CAD build for the part. Positions are in the model's coordinates, mm. A direction names the side the tool comes from. Round coordinates to 2 decimals unless told otherwise and drop trailing zeros. Order: outer loops, then holes, each group sorted by start corner. A loop starts at its lowest first (then second) coordinate and runs counter-clockwise, first axis right, second up. Notation, with made-up numbers: (67.25, 49.25) - (75.25, 49.25) arc R21 ccw to (75.25, 66.25) - close; hole circle Ø8 at (29.25, -20). An arc over 180 degrees is marked (long way). Write item = value, one per line.
from build123d import *

# Parameters (mm, degrees)
SKETCH1_W           = 67.3
SKETCH1_H           = 135.4
BOSS_EXTRUDE1_DEPTH = 15.1
FILLET1_R           = 5
FILLET2_R           = 3.75
SKETCH2_W           = 12.2
SKETCH2_H           = 4.45
CUT_EXTRUDE1_DEPTH  = 6
SKETCH3_W           = 8.2
SKETCH3_H           = 3.5
SKETCH3_W_2         = 8
SKETCH3_H_2         = 3.3
CUT_EXTRUDE2_DEPTH  = 3
FILLET3_R           = 3.75
SKETCH4_W           = 8
SKETCH4_H           = 3.3
BOSS_EXTRUDE2_DEPTH = 0.5
FILLET4_R           = 0.2
FILLET5_R           = 0.2
BOSS_EXTRUDE3_DEPTH = 2.1


with BuildPart() as part:
    # Sketch1 → Boss-Extrude1 (new body)
    with BuildSketch(Plane(origin=(0, 0, 0), x_dir=(1, 0, 0), z_dir=(0, 1, 0))):
        with Locations((33.65, 67.7)):
            Rectangle(SKETCH1_W, SKETCH1_H)
    extrude(amount=BOSS_EXTRUDE1_DEPTH)

    # Fillet1
    fillet1_edges = [part.edges().sort_by_distance(p)[0] for p in [
        (0, 7.55, -135.4),
        (67.3, 7.55, -135.4),
        (67.3, 7.55, 0),
        (0, 7.55, 0),
    ]]
    fillet(fillet1_edges, radius=FILLET1_R)

    # Fillet2
    fillet2_edges = [part.edges().sort_by_distance(p)[0] for p in [
        (0, 15.1, -67.7),
        (33.65, 15.1, -135.4),
        (33.65, 15.1, 0),
        (67.3, 15.1, -67.7),
        (1.464466094, 15.1, -1.464466094),
        (65.835533906, 15.1, -1.464466094),
        (65.835533906, 15.1, -133.935533906),
        (1.464466094, 15.1, -133.935533906),
    ]]
    fillet(fillet2_edges, radius=FILLET2_R)

    # Sketch2 → Cut-Extrude1 (cut)
    with BuildSketch(Plane.XY):
        with Locations((17.1, 8.125)):
            Rectangle(SKETCH2_W, SKETCH2_H)
        with Locations((50.2, 8.125)):
            Rectangle(SKETCH2_W, SKETCH2_H)
        with BuildLine():
            Line((30.7, 7.45), (36.6, 7.45))
            ThreePointArc((36.6, 7.45), (37.448528137, 7.801471863), (37.8, 8.65))
            Line((37.8, 8.65), (37.8, 9.15))
            ThreePointArc((37.8, 9.15), (37.448528137, 9.998528137), (36.6, 10.35))
            Line((36.6, 10.35), (30.7, 10.35))
            ThreePointArc((30.7, 10.35), (29.851471863, 9.998528137), (29.5, 9.15))
            Line((29.5, 9.15), (29.5, 8.65))
            ThreePointArc((29.5, 8.65), (29.851471863, 7.801471863), (30.7, 7.45))
        make_face()
    extrude(amount=-CUT_EXTRUDE1_DEPTH, mode=Mode.SUBTRACT)

    # Sketch3 → Cut-Extrude2 (cut)
    with BuildSketch(Plane(origin=(67.3, 0, 0), x_dir=(0, 0, -1), z_dir=(1, 0, 0))):
        with Locations((15.6, 7.6)):
            Rectangle(SKETCH3_W, SKETCH3_H)
        with Locations((15.6, 7.6)):
            Rectangle(SKETCH3_W_2, SKETCH3_H_2, mode=Mode.SUBTRACT)
    extrude(amount=-CUT_EXTRUDE2_DEPTH, mode=Mode.SUBTRACT)

    # Fillet3
    fillet3_edges = [part.edges().sort_by_distance(p)[0] for p in [
        (0, 0, -67.7),
        (33.65, 0, -135.4),
        (67.3, 0, -67.7),
        (33.65, 0, 0),
        (1.464466094, 0, -1.464466094),
        (65.835533906, 0, -1.464466094),
        (65.835533906, 0, -133.935533906),
        (1.464466094, 0, -133.935533906),
    ]]
    fillet(fillet3_edges, radius=FILLET3_R)

    # Sketch4 → Boss-Extrude2 (add)
    with BuildSketch(Plane(origin=(67.3, 0, 0), x_dir=(0, 0, -1), z_dir=(1, 0, 0))):
        with Locations((15.6, 7.6)):
            Rectangle(SKETCH4_W, SKETCH4_H)
    extrude(amount=BOSS_EXTRUDE2_DEPTH)

    # Fillet4
    fillet4_edges = [part.edges().sort_by_distance(p)[0] for p in [
        (66.05, 9.25, -11.6),
        (66.05, 9.25, -19.6),
        (66.05, 5.95, -19.6),
        (66.05, 5.95, -11.6),
    ]]
    fillet(fillet4_edges, radius=FILLET4_R)

    # Fillet5
    fillet5_edges = [part.edges().sort_by_distance(p)[0] for p in [
        (67.8, 7.6, -11.6),
        (67.8, 5.95, -15.6),
        (67.8, 7.6, -19.6),
        (67.8, 9.25, -15.6),
        (67.8, 9.191421356, -11.658578644),
        (67.8, 9.191421356, -19.541421356),
        (67.8, 6.008578644, -19.541421356),
        (67.8, 6.008578644, -11.658578644),
    ]]
    fillet(fillet5_edges, radius=FILLET5_R)

    # Sketch5 → Boss-Extrude3 (add)
    with BuildSketch(Plane.XY.offset(-6)):
        with BuildLine():
            Line((30.74, 8.35), (36.56, 8.35))
            ThreePointArc((36.56, 8.35), (36.941837662, 8.508162338), (37.1, 8.89))
            Line((37.1, 8.89), (37.1, 8.91))
            ThreePointArc((37.1, 8.91), (36.941837662, 9.291837662), (36.56, 9.45))
            Line((36.56, 9.45), (30.74, 9.45))
            ThreePointArc((30.74, 9.45), (30.358162338, 9.291837662), (30.2, 8.91))
            Line((30.2, 8.91), (30.2, 8.89))
            ThreePointArc((30.2, 8.89), (30.358162338, 8.508162338), (30.74, 8.35))
        make_face()
    extrude(amount=BOSS_EXTRUDE3_DEPTH)


solid = part.part
(1) Probe line 1 along X through (y, z) = (11.5, -82); line 2 along Z through (x, y) = (30.5, 3.5); line 3 along Z through (x, y) = (22, 6.5). List the from-to ranges inside material, lowest first.
Solved:
line_1 = 0 to 67.3
line_2 = -135.39 to -0.01
line_3 = -135.4 to -6
(2) Band-saw the part on B-B on x = 21. List the corners of the cut face in (y, z), plus the area to 3 significant figures.
Solved:
outline = (0, -131.65) arc R3.75 ccw to (3.75, -135.4) - (11.35, -135.4) arc R3.75 ccw to (15.1, -131.65) - (15.1, -3.75) arc R3.75 ccw to (11.35, 0) - (10.35, 0) - (10.35, -6) - (5.9, -6) - (5.9, 0) - (3.75, 0) arc R3.75 ccw to (0, -3.75) - close
area = 2,010 mm²
(3) Drop flat-ended pins along their axis: pin 1 (1.3 mm diameter, centred on y = 7.5, z = -2.5, fed in from -X); pin 2 (6 mm diameter, centred on x = 20.5, y = 7.5, fed in from +Z); pin 3 (3 mm diameter, centred on x = 66.5, y = 7.5, fed in from +Z); pin 4 (1.3 mm diameter, centred on x = 16.5, y = 8, fed in from +Z). Give the stop position or say it passes through.
Solved:
pin_1 = 0.35
pin_2 = 0
pin_3 = -0.79
pin_4 = -6
(4) Band-saw the part on A-A on z = -17. List the corners of the cut face in (x, y).
Solved:
outline = (0, 3.75) arc R3.75 ccw to (3.75, 0) - (63.55, 0) arc R3.75 ccw to (67.3, 3.75) - (67.3, 5.85) - (64.3, 5.85) - (64.3, 5.95) - (67.6, 5.95) arc R0.2 ccw to (67.8, 6.15) - (67.8, 9.05) arc R0.2 ccw to (67.6, 9.25) - (64.3, 9.25) - (64.3, 9.35) - (67.3, 9.35) - (67.3, 11.35) arc R3.75 ccw to (63.55, 15.1) - (3.75, 15.1) arc R3.75 ccw to (0, 11.35) - close
(5) Band-saw the part on C-C on z = -66. List the corners of the cut face in (x, y).
Solved:
outline = (0, 3.75) arc R3.75 ccw to (3.75, 0) - (63.55, 0) arc R3.75 ccw to (67.3, 3.75) - (67.3, 11.35) arc R3.75 ccw to (63.55, 15.1) - (3.75, 15.1) arc R3.75 ccw to (0, 11.35) - close
(6) Tool access for faces 1 (the flat face through (44.1, 8, -3)), 2 (the flat face through (0, 7, -67)): list every direction of +Z, -Z, +X, -X, +Y, -Y with a clear straight run to the whole face (end or side of a thin tool).
Solved:
face_1 = +Z
face_2 = +Z, -Z, -X, +Y, -Y
